```python
from build123d import *

# Parameters (mm, degrees)
F0_W     = 91.44
F0_H     = 17.78
F1_DEPTH = 25.4
F2_W     = 25.4
F2_H     = 25.4
F3_DEPTH = 50.8
F4_W     = 25.4
F4_H     = 50.8
F5_DEPTH = 43.18
F7_DEPTH = 15.24
F8_W     = 50.8
F8_H     = 50.8
F9_DEPTH = 17.78


with BuildPart() as f1:
    # F0 (on Right) → F1 (new body)
    with BuildSketch(Plane.YZ):
        with Locations((-32.5557654617, 24.2135534063)):
            Rectangle(F0_W, F0_H)
    extrude(amount=F1_DEPTH)

    # F2 (on face) → F3 (join)
    with BuildSketch(Plane(origin=(0, 0, 15.3235534063), x_dir=(1, 0, 0), z_dir=(0, 0, -1))):
        with Locations((12.7, -0.4642345383)):
            Rectangle(F2_W, F2_H)
    extrude(amount=F3_DEPTH)

    # F4 (on face) → F5 (join)
    with BuildSketch(Plane(origin=(0, 13.1642345383, 0), x_dir=(-1, 0, 0), z_dir=(0, 1, 0))):
        with Locations((-12.7, -10.0764465937)):
            Rectangle(F4_W, F4_H)
    extrude(amount=F5_DEPTH)

    # F6 (on face) → F7 (join)
    with BuildSketch(Plane(origin=(0, 0, 0), x_dir=(0, -1, 0), z_dir=(-1, 0, 0))):
        Polygon((12.2357654617, 15.3235534063), (-13.1642345383, 15.3235534063), (-56.3442345383, 15.3235534063), (-56.3442345383, -35.4764465937), (12.2357654617, -35.4764465937), align=None)
    extrude(amount=F7_DEPTH)

    # F8 (on face) → F9 (join)
    with BuildSketch(Plane(origin=(-15.24, 0, 0), x_dir=(0, -1, 0), z_dir=(-1, 0, 0))):
        with Locations((-13.1642345383, -10.0764465937)):
            Rectangle(F8_W, F8_H)
    extrude(amount=F9_DEPTH)


solid = f1.part
```
For this review, take the finished solid that the model builds, in its own axes (mm). A direction names the side the tool comes from. Coordinates: 2 decimals unless noted, no trailing zeros. Loops run counter-clockwise (first coordinate to the right, second up) from the corner with the lowest first, then second, coordinate; pieces in that order, holes last.
1. Add section A-A, the plane x = 11. Give the boundary of the cut face in (y, z).
2. Add section B-B, the plane y = -9.5. Give the boundary of the cut face in (x, z), then the cut area to 3 significant figures.
3. For line 1 (Z direction, x = 7, y = 50.5); line 2 (Y direction, x = -3, z = 12); line 3 (X direction, y = -42.5, z = 15.5), list the stretches that pass through material, from the lowest coordinate up.
4. Add section D-D, the plane x = -11. Give the boundary of the cut face in (y, z), then the cut area to 3 significant figures.
5. Add section C-C, the plane z = -12. Give the boundary of the cut face in (x, y), then the cut area to 3 significant figures.
6. Insertion check: P1, Ø6, axis at x = 8.5, z = -28, coming from the -Y side; P2, Ø14, axis at y = 47, z = 2, coming from the -X side; P3, Ø5.5, axis at x = 19, z = 28.5, coming from the +Y side. Each pin has a flat end and moves straight along its axis. Give the tip position at first contact, or say it passes through.
7. For faces 1 (the flat face through (-15.24, 48, -10)), 2 (the flat face through (13, -46, 15.324)), 3 (the flat face through (13, 13.164, 24)), 4 (the flat face through (0, -33, 24)), 5 (the flat face through (13, -33, 33.104)), list the 3-axis set-ups (+Z, -Z, +X, -X, +Y, -Y) from which the entire face can be reached by the end or side of a thin tool; tool diameter is ignored.
8. Mouldability with a two-part tool opening along Y and no side actions: class faces 6 (the flat face through (-24, 38.564, -10)), 7 (the flat face through (-3, -12.236, -10)), 8 (the flat face through (-3, 23, -35.476)) as +Y half, -Y half, draft (parallel to the pull), parting line (faces both ways), or undercut.
Result:
1. outline: (-78.28, 15.32) - (-12.24, 15.32) - (-12.24, -35.48) - (56.34, -35.48) - (56.34, 15.32) - (13.16, 15.32) - (13.16, 33.1) - (-78.28, 33.1) - close
2. outline: (-33.02, -35.48) - (25.4, -35.48) - (25.4, 33.1) - (0, 33.1) - (0, 15.32) - (-33.02, 15.32) - close
2. area: 3,420 mm2
3. line 1: z = -35.48 to 15.32
3. line 2: y = -12.24 to 56.34
3. line 3: x = 0 to 25.4
4. outline: (-12.24, -35.48) - (56.34, -35.48) - (56.34, 15.32) - (-12.24, 15.32) - close
4. area: 3,480 mm2
5. outline: (-33.02, -12.24) - (25.4, -12.24) - (25.4, 56.34) - (-15.24, 56.34) - (-15.24, 38.56) - (-33.02, 38.56) - close
5. area: 3,690 mm2
6. P1: stops at y = -12.24
6. P2: stops at x = -15.24
6. P3: stops at y = 13.16
7. face 1: +Z, -Z, -X, +Y
7. face 2: -Z, +X, -X, -Y
7. face 3: +Z, +X, -X, +Y
7. face 4: +Z, -X, +Y, -Y
7. face 5: +Z, +X, -X, +Y, -Y
8. face 6: +Y half
8. face 7: -Y half
8. face 8: draft
